Input: part model. Units: mm. Frame: model coordinates. A direction names the side the tool comes from. Coordinates: 2 decimals unless noted, no trailing zeros. Order: outer loops, then holes, each group sorted by start corner. A loop starts at its lowest first (then second) coordinate and runs counter-clockwise, first axis right, second up. Notation, with made-up numbers: (7.25, 37) -> (46.25, 37) arc R24 cw to (46.25, 73) -> close; hole circle Ø7 at (7, 85). An arc over 180 degrees is marked (long way). Use one line per item in the form item = value. Start each with the question number.
1) Access query for faces 4 (the flat face through (49, 109, -39)), 5 (the flat face through (48, 109, -2)), 6 (the flat face through (98.2, 0, -25.4)), 7 (the flat face through (48, -0.737, 12)). Directions: +Z, -Z, +X, -X, +Y, -Y. A direction counts if a zero-diameter tool reaches every point of the face in a straight line with its end or side. Return the directions, or none.
2) Ray query, line 1 along Z through (x, y) = (53, 152); line 2 along Y through (x, z) = (70, -38); line 3 along X through (y, z) = (128, -36.5). Return the intervals inside material, ascending.
3) Section query C-C on x = 93. Output: boundary loops of the cut face in (y, z), then the cut area to 3 significant figures.
4) Pin query (flat end, axial travel): pin 1 (1 mm diameter, centred on x = 87.5, y = 180.5, fed in from -Z); pin 2 (2 mm diameter, centred on y = -1.5, z = -52.5, fed in from +X); pin 3 (10 mm diameter, centred on x = 66.5, y = 33, fed in from +Z). Return the tip coordinate at first contact, or that it passes through.
5) Section query A-A on y = 139.69. Output: boundary loops of the cut face in (x, z), then the cut area to 3 significant figures.
6) Section query B-B on x = 10. Output: boundary loops of the cut face in (y, z).
7) Draft query along X for faces 1 (the flat face through (100, 109, -19)), 2 (the flat face through (48, 109, -37)), 3 (the cylindrical face through (11.34, 141.8, -37.99)). Return one class per face: pulls with the +X half, pulls with the -X half, needs draft (parallel to the pull), parting line crosses it, or undercut.
8) Section query D-D on y = 199.69. Output: boundary loops of the cut face in (x, z).
from build123d import *

# Parameters (mm, degrees)
SKETCH1_W                    = 100
SKETCH1_H                    = 214.69
BASE_FLANGE1_DEPTH           = 2
EDGE_FLANGE1_STRIP_W         = 9.4732
EDGE_FLANGE1_STRIP_H         = 2
EDGE_FLANGE1_STRIP_CUT_DEPTH = 214.69
EDGE_FLANGE1_DEPTH           = 214.69
EDGE_FLANGE2_STRIP_W         = 9.4732
EDGE_FLANGE2_STRIP_H         = 2
EDGE_FLANGE2_STRIP_CUT_DEPTH = 214.69
EDGE_FLANGE2_DEPTH           = 214.69
EDGE_FLANGE3_DEPTH           = 97.2634
EDGE_FLANGE3_BEND_DEPTH      = 97.2634
SKETCH18_W                   = 29
SKETCH18_H                   = 2.7366
SKETCH18_W_2                 = 27
CUT_EXTRUDE1_DEPTH           = 25
CUT_EXTRUDE2_REACH           = 246.818
SKETCH19_R                   = 2.5


# Sheet-metal steps are written as plain solids
with BuildPart() as part:
    # Sketch1 → Base-Flange1 (new body)
    with BuildSketch(Plane.XY):
        with Locations((50, 107.345)):
            Rectangle(SKETCH1_W, SKETCH1_H)
    extrude(amount=-BASE_FLANGE1_DEPTH)

    # Edge-Flange1 strip (across the edge) → Edge-Flange1 strip cut (cut)
    with BuildSketch(Plane(origin=(100, 214.69, -2), x_dir=(-1, 0, 0), z_dir=(0, -1, 0))):
        with Locations((-2, -1)):
            Rectangle(EDGE_FLANGE1_STRIP_W, EDGE_FLANGE1_STRIP_H)
    extrude(amount=EDGE_FLANGE1_STRIP_CUT_DEPTH, mode=Mode.SUBTRACT)

    # Edge-Flange1 section (across the edge) → Edge-Flange1 (add)
    with BuildSketch(Plane(origin=(100, 214.69, -2), x_dir=(-1, 0, 0), z_dir=(0, -1, 0))):
        with BuildLine():
            Line((0, 0.7366), (0, 37))
            Line((0, 37), (2, 37))
            Line((2, 37), (2, 0.7366))
            ThreePointArc((2, 0.7366), (2.215745145, 0.215745145), (2.7366, 0))
            Line((2.7366, 0), (2.7366, -2))
            ThreePointArc((2.7366, -2), (0.801531583, -1.198468417), (0, 0.7366))
        make_face()
    extrude(amount=EDGE_FLANGE1_DEPTH)

    # Edge-Flange2 strip (across the edge) → Edge-Flange2 strip cut (cut)
    with BuildSketch(Plane(origin=(98, 214.69, -39), x_dir=(0, 0, 1), z_dir=(0, -1, 0))):
        with Locations((-2, -1)):
            Rectangle(EDGE_FLANGE2_STRIP_W, EDGE_FLANGE2_STRIP_H)
    extrude(amount=EDGE_FLANGE2_STRIP_CUT_DEPTH, mode=Mode.SUBTRACT)

    # Edge-Flange2 section (across the edge) → Edge-Flange2 (add)
    with BuildSketch(Plane(origin=(98, 214.69, -39), x_dir=(0, 0, 1), z_dir=(0, -1, 0))):
        with BuildLine():
            Line((0, 0.7366), (0, 98))
            Line((0, 98), (2, 98))
            Line((2, 98), (2, 0.7366))
            ThreePointArc((2, 0.7366), (2.215745145, 0.215745145), (2.7366, 0))
            Line((2.7366, 0), (2.7366, -2))
            ThreePointArc((2.7366, -2), (0.801531583, -1.198468417), (0, 0.7366))
        make_face()
    extrude(amount=EDGE_FLANGE2_DEPTH)

    # Edge-Flange3 section (across the edge) → Edge-Flange3 (add)
    with BuildSketch(Plane(origin=(0, -0.7366, 0), x_dir=(0, 1, 0), z_dir=(1, 0, 0))):
        with BuildLine():
            Line((-2, 0.7366), (-2, 23))
            Line((-2, 23), (0, 23))
            Line((0, 23), (0, 0.7366))
            ThreePointArc((0, 0.7366), (0.215745145, 0.215745145), (0.7366, 0))
            Line((0.7366, 0), (0.7366, -2))
            ThreePointArc((0.7366, -2), (-1.198468417, -1.198468417), (-2, 0.7366))
        make_face()
    extrude(amount=EDGE_FLANGE3_DEPTH)

    # Edge-Flange3 section 2 (across the edge) → Edge-Flange3 bend (add)
    with BuildSketch(Plane(origin=(97.2634, -0.7366, -39), x_dir=(0, 1, 0), z_dir=(-1, 0, 0))):
        with BuildLine():
            Line((-2, 0.7366), (-2, 23))
            Line((-2, 23), (0, 23))
            Line((0, 23), (0, 0.7366))
            ThreePointArc((0, 0.7366), (0.215745145, 0.215745145), (0.7366, 0))
            Line((0.7366, 0), (0.7366, -2))
            ThreePointArc((0.7366, -2), (-1.198468417, -1.198468417), (-2, 0.7366))
        make_face()
    extrude(amount=EDGE_FLANGE3_BEND_DEPTH)

    # Sketch18 → Cut-Extrude1 (cut)
    with BuildSketch(Plane(origin=(0, -57.7366, -62), x_dir=(1, 0, 0), z_dir=(0, 0, 1))):
        with Locations((82.7634, 56.3683)):
            Rectangle(SKETCH18_W, SKETCH18_H)
        with Locations((13.5, 56.3683)):
            Rectangle(SKETCH18_W_2, SKETCH18_H)
    extrude(amount=CUT_EXTRUDE1_DEPTH, mode=Mode.SUBTRACT)

    # Cut-Extrude2: up to this face of the body (flat: up to its plane)
    cut_extrude2_end = Plane(part.part.faces().sort_by_distance((48.6317, 107.345, -39))[0])
    # Sketch19 → Cut-Extrude2 (cut, up to the picked face)
    with BuildSketch(Plane.XY, mode=Mode.PRIVATE) as cut_extrude2_sk1:
        with Locations((40, 199.69)):
            Circle(SKETCH19_R)
    cut_extrude2_tool1 = split(extrude(cut_extrude2_sk1.sketch, amount=-CUT_EXTRUDE2_REACH, mode=Mode.PRIVATE), bisect_by=cut_extrude2_end, keep=Keep.BOTH, mode=Mode.PRIVATE)
    # Sketch19 → Cut-Extrude2 (cut, up to the picked face)
    with BuildSketch(Plane.XY, mode=Mode.PRIVATE) as cut_extrude2_sk2:
        with Locations((10, 139.69)):
            Circle(SKETCH19_R)
    cut_extrude2_tool2 = split(extrude(cut_extrude2_sk2.sketch, amount=-CUT_EXTRUDE2_REACH, mode=Mode.PRIVATE), bisect_by=cut_extrude2_end, keep=Keep.BOTH, mode=Mode.PRIVATE)
    # Sketch19 → Cut-Extrude2 (cut, up to the picked face)
    with BuildSketch(Plane.XY, mode=Mode.PRIVATE) as cut_extrude2_sk3:
        with Locations((70, 139.69)):
            Circle(SKETCH19_R)
    cut_extrude2_tool3 = split(extrude(cut_extrude2_sk3.sketch, amount=-CUT_EXTRUDE2_REACH, mode=Mode.PRIVATE), bisect_by=cut_extrude2_end, keep=Keep.BOTH, mode=Mode.PRIVATE)
    add(cut_extrude2_tool1.solids().sort_by(Axis((40, 199.69, 0), (0, 0, -1)))[0], mode=Mode.SUBTRACT)
    add(cut_extrude2_tool2.solids().sort_by(Axis((10, 139.69, 0), (0, 0, -1)))[0], mode=Mode.SUBTRACT)
    add(cut_extrude2_tool3.solids().sort_by(Axis((70, 139.69, 0), (0, 0, -1)))[0], mode=Mode.SUBTRACT)


solid = part.part
Answers below:
q1.face_4 = -Z, +X, -X, +Y
q1.face_5 = -X, +Y, -Y
q1.face_6 = -Z, +X, -Y
q1.face_7 = +Z, +X, -X, +Y
q2.line_1 = -39 to -37, -2 to 0
q2.line_2 = 0 to 137.19, 142.19 to 214.69
q2.line_3 = 97.96 to 99.99
q3.outline = (-2.74, 0.74) arc R2.74 ccw to (0, -2) -> (214.69, -2) -> (214.69, 0) -> (0, 0) arc R0.74 cw to (-0.74, 0.74) -> (-0.74, 23) -> (-2.74, 23) -> close; (0, -39) -> (214.69, -39) -> (214.69, -37) -> (0, -37) -> close
q3.area = 909 mm^2
q4.pin_1 = -39
q4.pin_2 = 68.26
q4.pin_3 = 0
q5.outline = (0, -39) -> (7.5, -39) -> (7.5, -37) -> (0, -37) -> close; (0, -2) -> (7.5, -2) -> (7.5, 0) -> (0, 0) -> close; (12.5, -39) -> (67.5, -39) -> (67.5, -37) -> (12.5, -37) -> close; (12.5, -2) -> (67.5, -2) -> (67.5, 0) -> (12.5, 0) -> close; (72.5, -39) -> (97.26, -39) arc R2.74 ccw to (100, -36.26) -> (100, -2.74) arc R2.74 ccw to (97.26, 0) -> (72.5, 0) -> (72.5, -2) -> (97.26, -2) arc R0.74 cw to (98, -2.74) -> (98, -36.26) arc R0.74 cw to (97.26, -37) -> (72.5, -37) -> close
q5.area = 427 mm^2
q6.outline = (-2.74, 0.74) arc R2.74 ccw to (0, -2) -> (137.19, -2) -> (137.19, 0) -> (0, 0) arc R0.74 cw to (-0.74, 0.74) -> (-0.74, 23) -> (-2.74, 23) -> close; (0, -39) -> (137.19, -39) -> (137.19, -37) -> (0, -37) -> close; (142.19, -39) -> (214.69, -39) -> (214.69, -37) -> (142.19, -37) -> close; (142.19, -2) -> (214.69, -2) -> (214.69, 0) -> (142.19, 0) -> close
q7.face_1 = pulls with the +X half
q7.face_2 = needs draft
q7.face_3 = undercut
q8.outline = (0, -39) -> (37.5, -39) -> (37.5, -37) -> (0, -37) -> close; (0, -2) -> (37.5, -2) -> (37.5, 0) -> (0, 0) -> close; (42.5, -39) -> (97.26, -39) arc R2.74 ccw to (100, -36.26) -> (100, -2.74) arc R2.74 ccw to (97.26, 0) -> (42.5, 0) -> (42.5, -2) -> (97.26, -2) arc R0.74 cw to (98, -2.74) -> (98, -36.26) arc R0.74 cw to (97.26, -37) -> (42.5, -37) -> close
